Work out the finished part from the listing and answer in its coordinate system (mm). Give positions to 0.01 mm unless a question says otherwise; leave off trailing zeros. Order: outer loops, then holes, each group sorted by start corner. A loop starts at its lowest first (then second) coordinate and runs counter-clockwise, first axis right, second up.
Autodesk Inventor part; units mm, degrees
ref_plane "YZ Plane" through (0, 0, 0) normal (1, 0, 0) x (0, 1, 0)
ref_plane "XZ Plane" through (0, 0, 0) normal (0, 1, 0) x (-1, 0, 0)
ref_plane "XY Plane" through (0, 0, 0) normal (0, 0, 1) x (1, 0, 0)
sketch "Sketch1" plane through (0, 0, 0) normal (0, 1, 0) x (-1, 0, 0)
  line L0 (0, 0) -> (-100, 0)
  line L1 (0, -489) -> (0, 0)
  line L2 (-30.25, -489) -> (-30.25, -439)
  line L3 (-30.25, -439) -> (-112.25, -439)
  line L4 (-112.25, -439) -> (-112.25, -489)
  line L5 (-142.5, -489) -> (-112.25, -489)
  line L6 (-30.25, -489) -> (0, -489)
  line L7 (-142.5, -489) -> (-142.5, -389)
  line L8 (-142.5, -389) -> (-100, -389)
  line L9 (-100, -389) -> (-100, 0)
  dimension "d0" = 82
  dimension "d1" = 100
  dimension "d2" = 489
  dimension "d3" = 30.25
  dimension "d4" = 50
  dimension "d5" = 50
extrude "Extrusion1" add sketch "Sketch1" along normal blind 6.5
properties part number "inner_brace_left"
1. The part is cut by section C-C (z = -316). Write down the section's boundary in (x, y).
Findings below:
outline: (0, 0) - (100, 0) - (100, 6.5) - (0, 6.5) - close
2. Given P1, Ø3, axis at x = 65.5, y = 4.5, coming from the -Z side; P2, Ø3, axis at y = 3.5, z = -224, coming from the +X side; P3, Ø1, axis at y = 3, z = -109, coming from the -X side, each flat-ended and moving along its own axis, determine where each tip first touches the part or whether it passes through.
Findings below:
P1: stops at z = -439
P2: stops at x = 100
P3: stops at x = 0
3. Straight lines are drawn through the part: probe 1 along Z at (x, y) = (132, 6); probe 2 along Z at (x, y) = (46.5, 4.75); probe 3 along X at (y, z) = (1.5, -186). For each, find the intervals that lie inside material, in ascending order.
Findings below:
probe 1: z = -489 to -389
probe 2: z = -439 to 0
probe 3: x = 0 to 100
4. The part is cut by section A-A (y = 4). Write down the section's boundary in (x, z), then the cut area to 4 significant figures.
Findings below:
outline: (0, -489) - (30.25, -489) - (30.25, -439) - (112.25, -439) - (112.25, -489) - (142.5, -489) - (142.5, -389) - (100, -389) - (100, 0) - (0, 0) - close
area: 49,050 mm2
5. The part is cut by section B-B (x = 124.5). Write down the section's boundary in (y, z), then the cut area to 3 significant figures.
Findings below:
outline: (0, -489) - (6.5, -489) - (6.5, -389) - (0, -389) - close
area: 650 mm2
